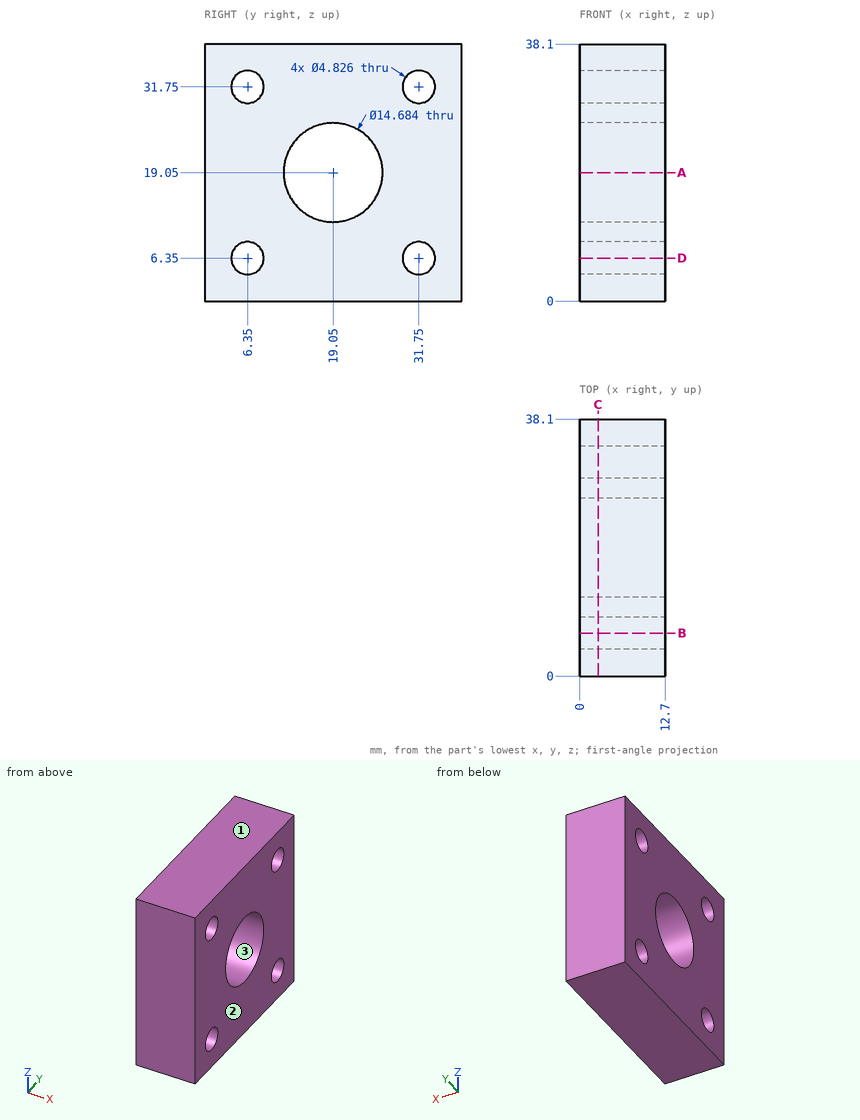
For this review, use the dimensioned drawing (mm, ordinates from the lowest corner) and the shaded views. Give positions to 0.01 mm unless a question says otherwise; leave off trailing zeros. Write each loop counter-clockwise with the first axis right and the second up, starting at its lowest first coordinate (ties: lowest second). Pieces come first, ordered by that corner, then holes. Notation, with made-up numbers: M 57.5,-2 L 68.5,-2 A12 cw 68.5,17 Z; hole C -36.5,44.25 d11. An arc over 180 degrees is marked long. Answer as a JSON object with one key per item and string values. Group by question number.
Item 1: For pin 1 Ø5 at (x, y) = (10.5, 13.5) entering from -Z; pin 2 Ø3 at (y, z) = (31.75, 6.35) entering from -X, all flat-tipped, find the tip position at first contact; note any pin that passes through.
Item 2: For probe 1 along Z at (x, y) = (9.5, 6.35); probe 2 along Y at (x, z) = (7.5, 5); probe 3 along Z at (x, y) = (7, 7.5), list the stretches that pass through material, from the lowest coordinate up. Write a range as [from, to].
Item 3: Consider section A-A on z = 19.05. Write out the cut boundary in (x, y).
Item 4: Draft analysis for pull direction Z (two halves, no side actions). For the marked faces 1, 2 and 3, state which applies: +Z half, -Z half, draft (parallel to the pull), parting line (faces both ways), or undercut.
Item 5: Consider section C-C on x = 2.75. Count the separate pieces of the cut face and the enclosed holes in it, plus the area to 3 significant figures.
Item 6: Consider section B-B on y = 6.35. Write out the cut boundary in (x, z).
Check result:
{
 "1": {"pin 1": "stops at z = 0", "pin 2": "passes through"},
 "2": {"probe 1": "z = [0, 3.94], [8.76, 29.34], [34.16, 38.1]", "probe 2": "y = [0, 4.35], [8.35, 29.75], [33.75, 38.1]", "probe 3": "z = [0, 4.23], [8.47, 29.63], [33.87, 38.1]"},
 "3": {"outline": "M 0,0 L 12.7,0 L 12.7,11.71 L 0,11.71 Z; M 0,26.39 L 12.7,26.39 L 12.7,38.1 L 0,38.1 Z"},
 "4": {"face 1": "+Z half", "face 2": "draft", "face 3": "undercut"},
 "5": {"separate pieces": "1", "enclosed holes": "5", "area": "1,210 mm^2"},
 "6": {"outline": "M 0,0 L 12.7,0 L 12.7,3.94 L 0,3.94 Z; M 0,8.76 L 12.7,8.76 L 12.7,29.34 L 0,29.34 Z; M 0,34.16 L 12.7,34.16 L 12.7,38.1 L 0,38.1 Z"}
}
